Job drawing, mm, ordinate dimensions from the low corner. One solid piece. Give positions to 0.01 mm unless a question says otherwise; leave off trailing zeros. Loops run counter-clockwise (first coordinate to the right, second up) from the corner with the lowest first, then second, coordinate; pieces in that order, holes last. Notation, with made-up numbers: M -15.75,-17.75 L -5.75,-17.75 A21 cw -5.75,2.25 Z; hole C 42.5,28.25 d7. An arc over 180 degrees is marked long. One line per question, with ' | ' between items.
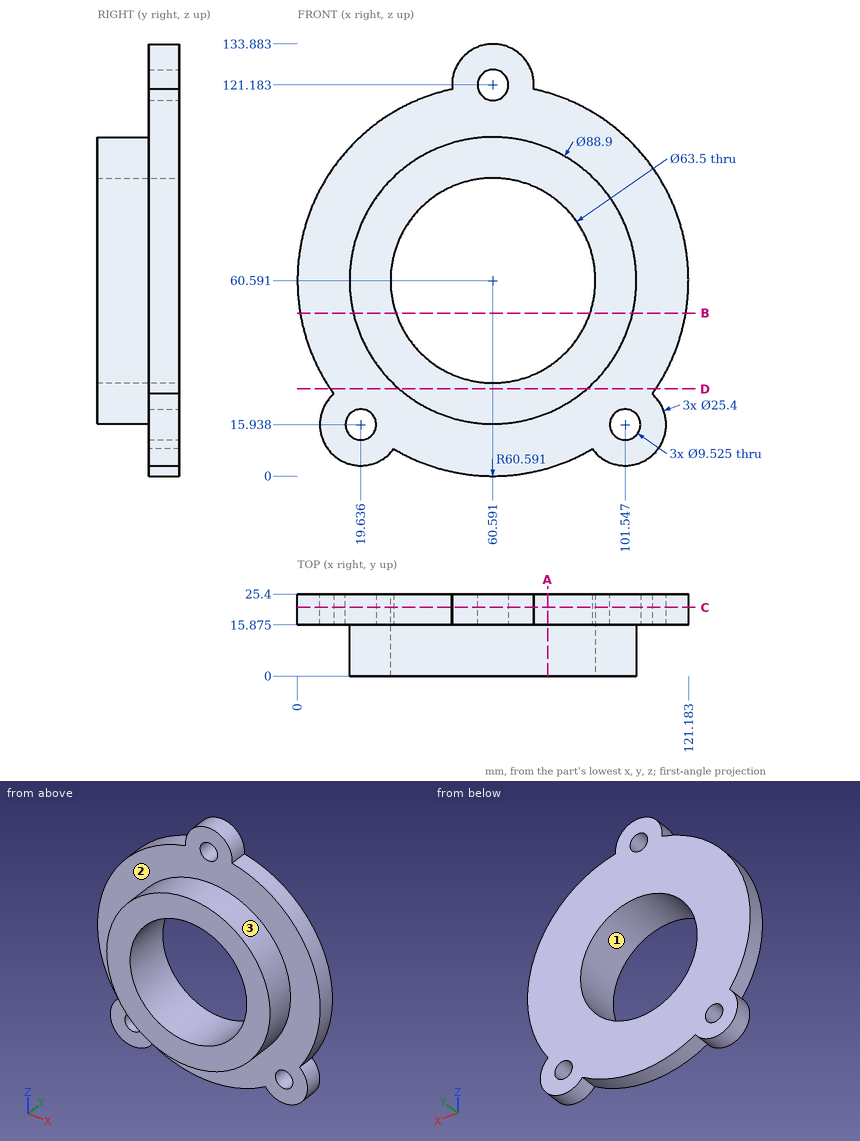
Item 1: Drill centre lines: line 1 along X through (y, z) = (24, 15.5) (1 decimal); line 2 along X through (y, z) = (11.75, 62); line 3 along Y through (x, z) = (109, 82.5) (1 decimal). Where is each one in solid material? Low to high. Write a range as [from, to].
Conclusion:
line 1: [6.9, 14.9], [24.4, 96.8], [106.3, 114.2] | line 2: [16.16, 28.87], [92.31, 105.02] | line 3: [15.9, 25.4]
Item 2: Saw through at A-A on x = 77.5. Give the cut face in (y, z) (1 decimal), and give its area (3 significant figures).
Conclusion:
outline: M 0,19.5 L 15.9,19.5 L 15.9,2.4 L 25.4,2.4 L 25.4,33.7 L 0,33.7 Z; M 0,87.5 L 25.4,87.5 L 25.4,118.8 L 15.9,118.8 L 15.9,101.7 L 0,101.7 Z | area: 1,050 mm²
Item 3: Mould opens along Z. For the marked faces 1, 2 and 3 say: pulls with the +Z half, pulls with the -Z half, needs draft (parallel to the pull), parting line crosses it, or undercut.
Conclusion:
face 1: undercut | face 2: needs draft | face 3: parting line crosses it
Item 4: Saw through at D-D on z = 27. Give the cut face in (x, y) (1 decimal).
Conclusion:
outline: M 10.2,15.9 L 31.5,15.9 L 31.5,0 L 89.7,0 L 89.7,15.9 L 111,15.9 L 111,25.4 L 10.2,25.4 Z
Item 5: Saw through at B-B on z = 50.5. Give the cut face in (x, y) (1 decimal).
Conclusion:
outline: M 0.8,15.9 L 17.3,15.9 L 17.3,0 L 30.5,0 L 30.5,25.4 L 0.8,25.4 Z; M 90.7,0 L 103.9,0 L 103.9,15.9 L 120.3,15.9 L 120.3,25.4 L 90.7,25.4 Z
Item 6: Drop flat-ended pins along their axis: P1, Ø6, axis at x = 60.5, z = 116.5, coming from the +Y side; P2, Ø8.5, axis at x = 101.55, z = 15.94, coming from the +Y side; P3, Ø5, axis at x = 53, y = 18, coming from the +Z side; P4, Ø8, axis at x = 67.5, y = 19.5, coming from the -Z side. Give the stop position or say it passes through.
Conclusion:
P1: y = 25.4 | P2: through | P3: z = 132.82 | P4: z = 0.07
Item 7: Saw through at C-C on y = 21.25. State how many separate pieces and enclosed holes the cut face has, and give its area (3 significant figures).
Conclusion:
separate pieces: 1 | enclosed holes: 4 | area: 8,950 mm²
